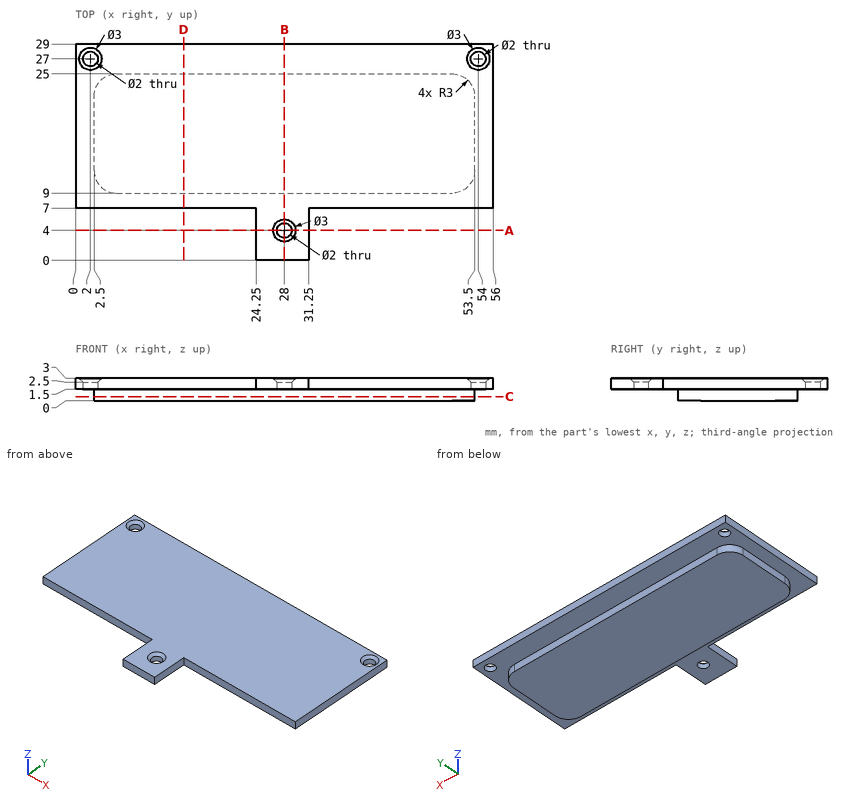
Check sheet for the drawn part. Datum: minimum x, y, z corner. Units: mm. Give positions to 0.01 mm unless a question says otherwise; leave off trailing zeros. Order: outer loops, then holes, each group sorted by start corner. A loop starts at its lowest first (then second) coordinate and runs counter-clockwise, first axis right, second up. Notation, with made-up numbers: (38.5, -2) - (73.5, -2) arc R23 cw to (73.5, 28) - close; hole circle Ø3 at (70.25, 30). An arc over 180 degrees is marked (long way). Answer as a JSON object with one key per item and string values.
(1) Cross-section at D-D (x = 14.5). Record the cut outline in (y, z).
Report:
{"outline": "(7, 1.5) - (9, 1.5) - (9, 0) - (25, 0) - (25, 1.5) - (29, 1.5) - (29, 3) - (7, 3) - close"}
(2) Cross-section at B-B (x = 28). Record the cut outline in (y, z), then the cut area to 4 significant figures.
Report:
{"outline": "(0, 1.5) - (3, 1.5) - (3, 2.5) - (2.5, 3) - (0, 3) - close; (5, 1.5) - (9, 1.5) - (9, 0) - (25, 0) - (25, 1.5) - (29, 1.5) - (29, 3) - (5.5, 3) - (5, 2.5) - close", "area": "64.25 mm^2"}
(3) Cross-section at C-C (z = 0.55). Record the cut outline in (x, y), then the cut area to 3 significant figures.
Report:
{"outline": "(2.5, 12) arc R3 ccw to (5.5, 9) - (50.5, 9) arc R3 ccw to (53.5, 12) - (53.5, 22) arc R3 ccw to (50.5, 25) - (5.5, 25) arc R3 ccw to (2.5, 22) - close", "area": "808 mm^2"}
(4) Cross-section at A-A (y = 4). Record the cut outline in (x, z), then the cut area to 3 significant figures.
Report:
{"outline": "(24.25, 1.5) - (27, 1.5) - (27, 2.5) - (26.5, 3) - (24.25, 3) - close; (29, 1.5) - (31.25, 1.5) - (31.25, 3) - (29.5, 3) - (29, 2.5) - close", "area": "7.25 mm^2"}
(5) Depth check by flat-ended pin: pin 1 Ø1.6 at (y, z) = (5, 2) entering from -X; pin 2 Ø1.6 at (y, z) = (19.5, 0.5) entering from +X; pin 3 Ø1.2 at (x, z) = (13.5, 2) entering from -Y. Enter the tip coordinate at first touch or a pass-through.
Report:
{"pin 1": "x = 24.25", "pin 2": "x = 53.5", "pin 3": "y = 7"}
(6) Material ranges on line 1 (X direction, y = 27, z = 1.9); line 2 (Y direction, x = 2, z = 1.95); line 3 (Y direction, x = 28, z = 2.35), recorded low to high.
Report:
{"line 1": "0 to 1, 3 to 53, 55 to 56", "line 2": "7 to 26, 28 to 29", "line 3": "0 to 3, 5 to 29"}
